```python
from build123d import *

# Parameters (mm, degrees)
SKETCH1_W            = 93
SKETCH1_H            = 44
BOSS_EXTRUDE1_DEPTH  = 8
SKETCH2_W            = 69
SKETCH2_H            = 36
CUT_EXTRUDE1_DEPTH   = 8
FILLET1_R            = 4
FILLET2_R            = 2
CUT_EXTRUDE2_START   = -9
CUT_EXTRUDE2_DEPTH   = 10
FILLET3_R            = 3
FILLET3_OF_MIRROR1_R = 3


with BuildPart() as part:
    # Sketch1 → Boss-Extrude1 (new body)
    with BuildSketch(Plane(origin=(0, 0, 0), x_dir=(1, 0, 0), z_dir=(0, 1, 0))):
        Rectangle(SKETCH1_W, SKETCH1_H)
    extrude(amount=BOSS_EXTRUDE1_DEPTH)

    # Sketch2 → Cut-Extrude1 (cut)
    with BuildSketch(Plane(origin=(0, 8, 0), x_dir=(1, 0, 0), z_dir=(0, 1, 0))):
        Rectangle(SKETCH2_W, SKETCH2_H)
    extrude(amount=-CUT_EXTRUDE1_DEPTH, mode=Mode.SUBTRACT)

    # Fillet1
    fillet1_edges = [part.edges().sort_by_distance(p)[0] for p in [
        (34.5, 4, 18),
        (-34.5, 4, 18),
        (-34.5, 4, -18),
        (34.5, 4, -18),
    ]]
    fillet(fillet1_edges, radius=FILLET1_R)

    # Fillet2
    fillet2_edges = [part.edges().sort_by_distance(p)[0] for p in [
        (-46.5, 4, -22),
        (46.5, 4, -22),
        (46.5, 4, 22),
        (-46.5, 4, 22),
    ]]
    fillet(fillet2_edges, radius=FILLET2_R)

    # Sketch3 → Cut-Extrude2 (cut)
    with BuildSketch(Plane(origin=(0, 8, 0), x_dir=(1, 0, 0), z_dir=(0, 1, 0)).offset(CUT_EXTRUDE2_START)):
        with BuildLine():
            Line((-38.5, 9.522429027), (-38.5, -9.522429027))
            ThreePointArc((-38.5, -9.522429027), (-41.652222577, -13.499394615), (-46.5, -15))
            Line((-46.5, -15), (-46.5, 15))
            ThreePointArc((-46.5, 15), (-41.652222577, 13.499394615), (-38.5, 9.522429027))
        make_face()
    cut_extrude2 = extrude(amount=CUT_EXTRUDE2_DEPTH, mode=Mode.SUBTRACT)

    # Fillet3
    fillet3_edges = [part.edges().sort_by_distance(p)[0] for p in [
        (-38.5, 4, -9.522429027),
        (-38.5, 4, 9.522429027),
    ]]
    fillet(fillet3_edges, radius=FILLET3_R)

    # Mirror1: Cut-Extrude2 across plane
    add(cut_extrude2.mirror(Plane(origin=(0, 0, 0), x_dir=(0, 0, 1), z_dir=(1, 0, 0))), mode=Mode.SUBTRACT)

    # Fillet3 of Mirror1
    fillet3_of_mirror1_edges = [part.edges().sort_by_distance(p)[0] for p in [
        (38.5, 4, -9.522429027),
        (38.5, 4, 9.522429027),
    ]]
    fillet(fillet3_of_mirror1_edges, radius=FILLET3_OF_MIRROR1_R)


solid = part.part
```
Can you work these out from the model? Positions are in its coordinate system, mm. A direction names the side the tool comes from. Give positions to 0.01 mm unless a question says otherwise; leave off trailing zeros. Loops run counter-clockwise (first coordinate to the right, second up) from the corner with the lowest first, then second, coordinate; pieces in that order, holes last. Notation, with made-up numbers: M 46,40.25 L 105,40.25 A9 cw 105,48.25 Z; hole C 7,84 d4. An arc over 180 degrees is marked long. Use one line per item in the form item = value. Start each with the question number.
(1) On a 3-axis mill with a long thin cutter (end or side, diameter ignored), from which of +Z, -Z, +X, -X, +Y, -Y can I reach the whole of each face in a straight line? I mean faces 4 (the cylindrical face through (-45.93, 4.06, 21.4)), 5 (the cylindrical face through (-33.297, 3.944, -16.859)), 6 (the flat face through (-38.5, 4, 0)), 7 (the flat face through (38.5, 4, 0)). Say none if no direction works.
(2) Please list where these lines run through material, in increasing order: line 1 (X direction, y = 1.25, z = -8.5); line 2 (Z direction, x = -29, y = 3.5); line 3 (X direction, y = 6.5, z = 17.5).
(3) I want a section at A-A, the plane z = 1.5. Write out the boundary of the cut face in (x, y).
(4) I want a section at B-B, the plane x = 2.5. Write out the boundary of the cut face in (y, z).
(5) I'm going to push flat-ended pins straight in: P1, Ø2.5, axis at y = 6, z = 3.5, coming from the -X side; P2, Ø4, axis at y = 5, z = 2, coming from the +X side; P3, Ø6, axis at x = 22, z = 12.5, coming from the -Y side. Where does each tip first touch, or does it pass through?
(6) I want a section at C-C, the plane y = 1.5. Write out the boundary of the cut face in (x, z).
(7) Thinking about a two-plate mould opening in Z: for faces 1 (the flat face through (46.5, 4, 18)), 2 (the flat face through (-1, 4, 22)), 3 (the flat face through (0, 4, -18)), which applies, released by +Z, released by -Z, zero draft, split by the parting line, or undercut?
Worked out:
q1.face_4 = +Z, -X, +Y, -Y
q1.face_5 = +Y, -Y
q1.face_6 = -X, +Y, -Y
q1.face_7 = +X, +Y, -Y
q2.line_1 = -38.5 to -34.5, 34.5 to 38.5
q2.line_2 = -22 to -18, 18 to 22
q2.line_3 = -46.5 to -32.44, 32.44 to 46.5
q3.outline = M -38.5,0 L -34.5,0 L -34.5,8 L -38.5,8 Z; M 34.5,0 L 38.5,0 L 38.5,8 L 34.5,8 Z
q4.outline = M 0,-22 L 8,-22 L 8,-18 L 0,-18 Z; M 0,18 L 8,18 L 8,22 L 0,22 Z
q5.P1 = -38.5
q5.P2 = 38.5
q5.P3 = through
q6.outline = M -46.5,-20 A2 ccw -44.5,-22 L 44.5,-22 A2 ccw 46.5,-20 L 46.5,-15 A8.58 cw 38.81,-10.23 A3 cw 38.5,-8.9 L 38.5,8.9 A3 cw 38.81,10.23 A8.58 cw 46.5,15 L 46.5,20 A2 ccw 44.5,22 L -44.5,22 A2 ccw -46.5,20 L -46.5,15 A8.58 cw -38.81,10.23 A3 cw -38.5,8.9 L -38.5,-8.9 A3 cw -38.81,-10.23 A8.58 cw -46.5,-15 Z; hole M -34.5,-14 A4 ccw -30.5,-18 L 30.5,-18 A4 ccw 34.5,-14 L 34.5,14 A4 ccw 30.5,18 L -30.5,18 A4 ccw -34.5,14 Z
q7.face_1 = zero draft
q7.face_2 = released by +Z
q7.face_3 = undercut
